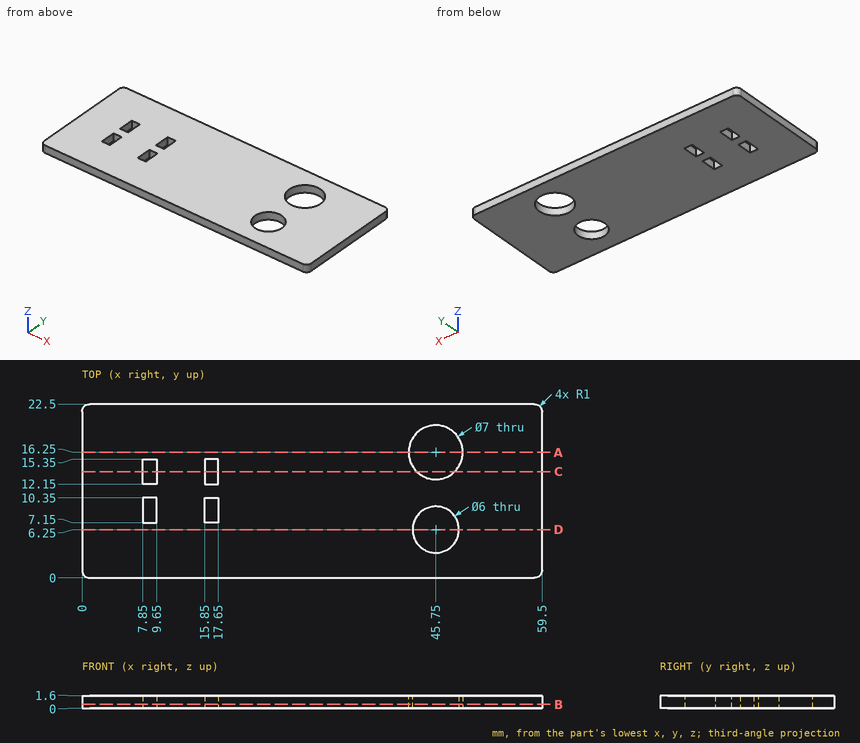
Study the drawing (mm; zero at the part's minimum x, y, z) and answer. Coordinates: 2 decimals unless noted, no trailing zeros. Loops run counter-clockwise (first coordinate to the right, second up) from the corner with the lowest first, then second, coordinate; pieces in that order, holes last. Notation, with made-up numbers: M 19,12 L 28,12 A26 ccw 28,49 Z; hole C -33,-36 d5. An arc over 180 degrees is marked long. Answer in a Markdown table with one row per item. Add a question column.
1. Find section A-A, the plane y = 16.25. Write down the section's boundary in (x, z).
2. Find section B-B, the plane z = 0.5. Write down the section's boundary in (x, y), then the cut area to 3 significant figures.
3. A flat-ended cylindrical pin translates along its axis: P1, Ø6.5, axis at x = 45.75, y = 16.25, coming from the -Z side. Find the tip coordinate at first contact, or state that the pin passes through.
4. Find section C-C, the plane y = 13.75. Write down the section's boundary in (x, z), then the cut area to 3 significant figures.
5. Consider L1, parallel to Y at x = 45.75, z = 0.6; L2, parallel to X at y = 14.25, z = 0.3; L3, parallel to Y at x = 9.5, z = 0.65. Determine where each line is inside the solid, lowest interval first.
6. Find section D-D, the plane y = 6.25. Write down the section's boundary in (x, z).
Reported:
| question | item | result |
|---|---|---|
| 1 | outline | M 0,0 L 42.25,0 L 42.25,1.6 L 0,1.6 Z; M 49.25,0 L 59.5,0 L 59.5,1.6 L 49.25,1.6 Z |
| 2 | outline | M 0,1 A1 ccw 1,0 L 58.5,0 A1 ccw 59.5,1 L 59.5,21.5 A1 ccw 58.5,22.5 L 1,22.5 A1 ccw 0,21.5 Z; hole M 7.85,7.15 L 9.65,7.15 L 9.65,10.35 L 7.85,10.35 Z; hole M 7.85,12.15 L 9.65,12.15 L 9.65,15.35 L 7.85,15.35 Z; hole M 15.85,7.15 L 17.65,7.15 L 17.65,10.35 L 15.85,10.35 Z; hole M 15.85,12.15 L 17.65,12.15 L 17.65,15.35 L 15.85,15.35 Z; hole C 45.75,16.25 d7; hole C 45.75,6.25 d6 |
| 2 | area | 1,250 mm^2 |
| 3 | P1 | passes through |
| 4 | outline | M 0,0 L 7.85,0 L 7.85,1.6 L 0,1.6 Z; M 9.65,0 L 15.85,0 L 15.85,1.6 L 9.65,1.6 Z; M 17.65,0 L 43.3,0 L 43.3,1.6 L 17.65,1.6 Z; M 48.2,0 L 59.5,0 L 59.5,1.6 L 48.2,1.6 Z |
| 4 | area | 81.6 mm^2 |
| 5 | L1 | y = 0 to 3.25, 9.25 to 12.75, 19.75 to 22.5 |
| 5 | L2 | x = 0 to 7.85, 9.65 to 15.85, 17.65 to 42.88, 48.62 to 59.5 |
| 5 | L3 | y = 0 to 7.15, 10.35 to 12.15, 15.35 to 22.5 |
| 6 | outline | M 0,0 L 42.75,0 L 42.75,1.6 L 0,1.6 Z; M 48.75,0 L 59.5,0 L 59.5,1.6 L 48.75,1.6 Z |
